Autodesk Inventor part; units mm, degrees
ref_plane "YZ Plane" through (0, 0, 0) normal (1, 0, 0) x (0, 1, 0)
ref_plane "XZ Plane" through (0, 0, 0) normal (0, 1, 0) x (-1, 0, 0)
ref_plane "XY Plane" through (0, 0, 0) normal (0, 0, 1) x (1, 0, 0)
sketch "Эскиз1" plane through (0, 0, 0) normal (0, 0, 1) x (1, 0, 0)
  line L0 (-36.8, -20) -> (36.8, -20)
  line L1 (36.8, -20) -> (36.8, 20)
  line L2 (36.8, 20) -> (-36.8, 20)
  line L3 (-36.8, 20) -> (-36.8, -20)
  line L4 (-36.8, -20) -> (36.8, 20) construction
  line L5 (36.8, -20) -> (-36.8, 20) construction
  line L6 (-17.8, -8) -> (-32.8, -8) construction
  line L7 (-32.8, -8) -> (-32.8, 8) construction
  line L8 (-32.8, 8) -> (-17.8, 8) construction
  line L9 (-17.8, 8) -> (-17.8, -8) construction
  line L10 (-17.8, -8) -> (-32.8, 8) construction
  line L11 (-32.8, -8) -> (-17.8, 8) construction
  circle A0 centre (-32.8, -8) radius 1.6
  circle A1 centre (-32.8, 8) radius 1.6
  circle A2 centre (-17.8, 8) radius 1.6
  circle A3 centre (-17.8, -8) radius 1.6
  line L12 (0, 0) -> (0, -20) construction
  line L13 (17.8, -8) -> (32.8, -8) construction
  line L14 (32.8, -8) -> (32.8, 8) construction
  line L15 (32.8, 8) -> (17.8, 8) construction
  line L16 (17.8, 8) -> (17.8, -8) construction
  line L17 (17.8, -8) -> (32.8, 8) construction
  line L18 (32.8, -8) -> (17.8, 8) construction
  circle A4 centre (32.8, -8) radius 1.6
  circle A5 centre (32.8, 8) radius 1.6
  circle A6 centre (17.8, 8) radius 1.6
  circle A7 centre (17.8, -8) radius 1.6
  point P0 (-25.3, 0)
  point P1 (25.3, 0)
  dimension "d0" = 73.6
  dimension "d1" = 40
  dimension "d2" = 15
  dimension "d3" = 16
  dimension "d4" = 4
  dimension "d5" = 3.2
  dimension "d6" = 3.2
  dimension "d7" = 3.2
  dimension "d8" = 3.2
  dimension "d9" = 20
extrude "Выдавливание1" add sketch "Эскиз1" along normal blind 4
sketch "Эскиз2" plane through (0, 0, 4) normal (0, 0, 1) x (1, 0, 0)
  line L0 (-12, 12.1) -> (12, 12.1) construction
  line L1 (-12, 7.2) -> (12, 7.2)
  line L2 (12, 17) -> (-12, 17)
  arc A0 (-12, 17) -> (-12, 7.2) centre (-12, 12.1) ccw
  arc A1 (12, 7.2) -> (12, 17) centre (12, 12.1) ccw
  line L3 (36.8, 20) -> (-36.8, 20)
  point P0 (0, 0)
  point P1 (0, 12.1)
  dimension "d12" = 12
  dimension "d13" = 9.8
  dimension "d14" = 3
extrude "Выдавливание2" cut sketch "Эскиз2" against normal blind 10
properties part number "стена_движения_каретки_з"
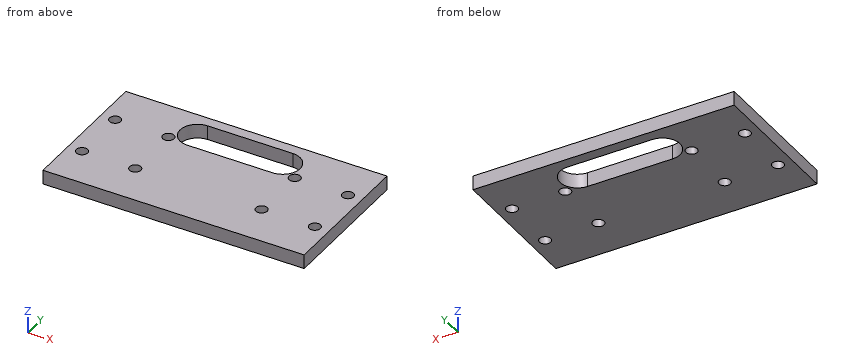
Can you work these out from the model? Positions are in its coordinate system, mm. Give positions to 0.01 mm unless a question says otherwise; leave off trailing zeros. Loops run counter-clockwise (first coordinate to the right, second up) from the corner with the lowest first, then second, coordinate; pieces in that order, holes last. Notation, with made-up numbers: M -14.5,-27 L 16.5,-27 A33 ccw 16.5,8 Z; hole C 35.5,13 d2. An arc over 180 degrees is marked long. One line per item, written item: value. Start each with the question number.
1) If we section it at D-D, the plane x = 4: Write out the boundary of the cut face in (y, z).
2) If we section it at A-A, the plane y = -8: Write out the boundary of the cut face in (x, z).
3) If we section it at B-B, the plane x = -32.8: Write out the boundary of the cut face in (y, z).
4) If we section it at C-C, the plane y = 12.1: Write out the boundary of the cut face in (x, z).
5) I'm going to push a flat-ended pin straight in: pin 1 (4 mm diameter, centred on x = 17.8, y = -8, fed in from +Z). Where does the tip first touch, or does it pass through?
6) If I drill on line 1 (Y direction, x = -17.8, z = 1.85); line 2 (Y direction, x = 10.5, z = 1.35); line 3 (X direction, y = 16, z = 0.2), over which ranges is the centre line in solid material (lowest first)? Write a range as [from, to].
Completed:
1. outline: M -20,0 L 7.2,0 L 7.2,4 L -20,4 Z; M 17,0 L 20,0 L 20,4 L 17,4 Z
2. outline: M -36.8,0 L -34.4,0 L -34.4,4 L -36.8,4 Z; M -31.2,0 L -19.4,0 L -19.4,4 L -31.2,4 Z; M -16.2,0 L 16.2,0 L 16.2,4 L -16.2,4 Z; M 19.4,0 L 31.2,0 L 31.2,4 L 19.4,4 Z; M 34.4,0 L 36.8,0 L 36.8,4 L 34.4,4 Z
3. outline: M -20,0 L -9.6,0 L -9.6,4 L -20,4 Z; M -6.4,0 L 6.4,0 L 6.4,4 L -6.4,4 Z; M 9.6,0 L 20,0 L 20,4 L 9.6,4 Z
4. outline: M -36.8,0 L -16.9,0 L -16.9,4 L -36.8,4 Z; M 16.9,0 L 36.8,0 L 36.8,4 L 16.9,4 Z
5. pin 1: stops at z = 4
6. line 1: y = [-20, -9.6], [-6.4, 6.4], [9.6, 20]
6. line 2: y = [-20, 7.2], [17, 20]
6. line 3: x = [-36.8, -14.97], [14.97, 36.8]
